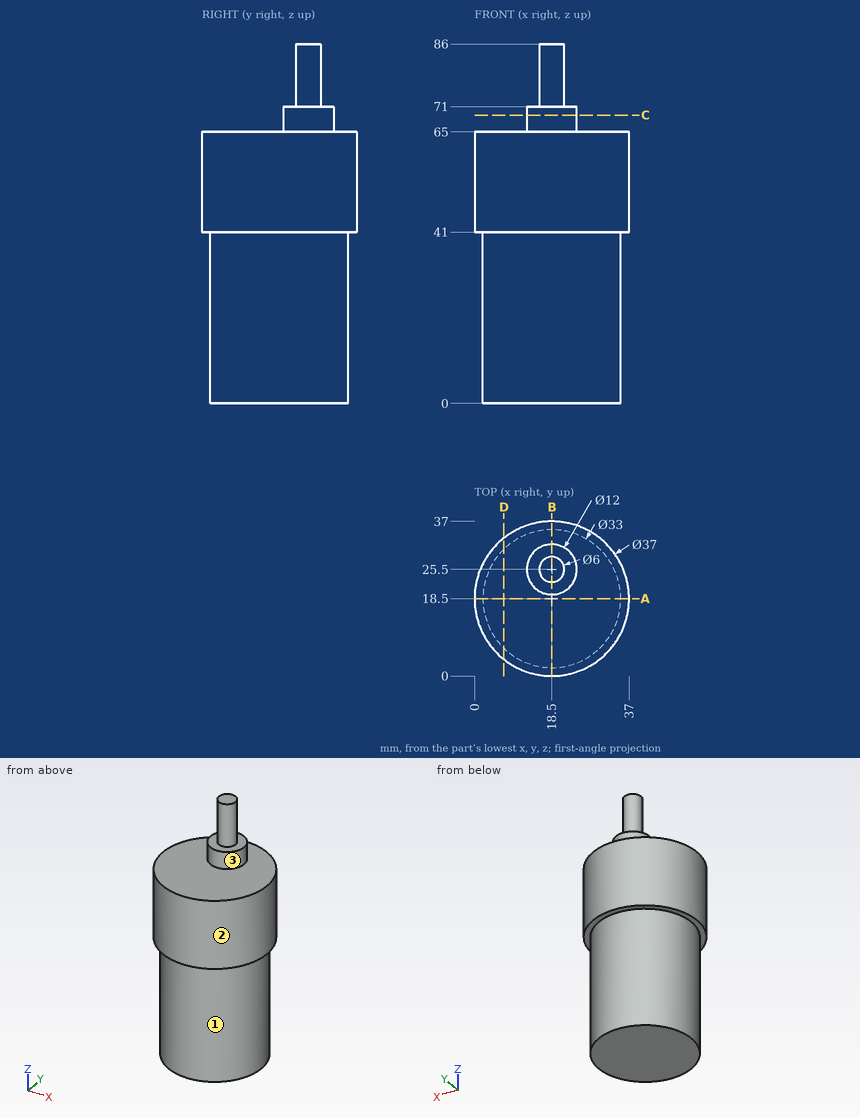
Could you check a few things on this drawing? It's one solid part, dimensions in mm from its lowest x, y, z. A direction names the side the tool comes from. Coordinates: 2 decimals unless noted, no trailing zeros. Write each loop counter-clockwise with the first axis right and the second up, starting at its lowest first coordinate (ties: lowest second). Pieces come first, ordered by that corner, then holes.
Q1. Imagine slicing it at D-D, the plane x = 7. List the corners of the cut face in (y, z) for me.
Results found:
outline: (4.01, 41) - (6.67, 41) - (6.67, 0) - (30.33, 0) - (30.33, 41) - (32.99, 41) - (32.99, 65) - (4.01, 65) - close
Q2. Imagine slicing it at A-A, the plane y = 18.5. List the corners of the cut face in (x, z) for me, plus the area to 3 significant figures.
Results found:
outline: (0, 41) - (2, 41) - (2, 0) - (35, 0) - (35, 41) - (37, 41) - (37, 65) - (0, 65) - close
area: 2,240 mm2
Q3. For P1, Ø1, axis at x = 18, z = 76.5, coming from the -Y side; P2, Ø1, axis at x = 29, z = 64.5, coming from the -Y side; P3, Ø18.5, axis at x = 10, y = 15, coming from the +Z side, each with a flat end and sliding along its axis, tell me the tip position at first contact or that it passes through.
Results found:
P1: stops at y = 22.5
P2: stops at y = 2.94
P3: stops at z = 71
Q4. Imagine slicing it at C-C, the plane z = 69. List the corners of the cut face in (x, y) for me.
Results found:
outline: circle Ø12 at (18.5, 25.5)
Q5. Imagine slicing it at B-B, the plane x = 18.5. List the corners of the cut face in (y, z) for me.
Results found:
outline: (0, 41) - (2, 41) - (2, 0) - (35, 0) - (35, 41) - (37, 41) - (37, 65) - (31.5, 65) - (31.5, 71) - (28.5, 71) - (28.5, 86) - (22.5, 86) - (22.5, 71) - (19.5, 71) - (19.5, 65) - (0, 65) - close
Q6. Please list where these lines run through material, in increasing order: L1, parallel to Z at x = 27, y = 19; L2, parallel to Z at x = 32, y = 29; L3, parallel to Y at x = 16.5, z = 70.5.
Results found:
L1: z = 0 to 65
L2: z = 41 to 65
L3: y = 19.84 to 31.16
Q7. Which directions (+Z, -Z, +X, -X, +Y, -Y) give clear straight access to the entire face, cutting with the end or side of a thin tool? Please do the marked faces 1, 2 and 3.
Results found:
face 1: -Z
face 2: +Z, -Z
face 3: +Z
